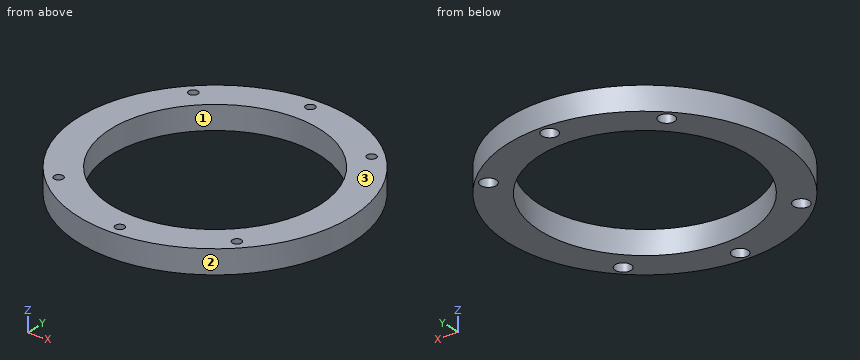
from build123d import *

# Parameters (mm, degrees)
CYLINDER057_R       = 87
CYLINDER057_DEPTH   = 15
CYLINDER058_R       = 66.5
CYLINDER058_DEPTH   = 15
HOLE019_D           = 5.8
HOLE019_DEPTH       = 25
HOLE019_CBORE_D     = 10
HOLE019_CBORE_DEPTH = 5.4


with BuildPart() as part:
    # Cylinder057 → Cylinder057 (join)
    with BuildSketch(Plane.XY):
        Circle(CYLINDER057_R)
    extrude(amount=CYLINDER057_DEPTH)

    # Cylinder058 → Cylinder058 (cut)
    with BuildSketch(Plane.XY):
        Circle(CYLINDER058_R)
    extrude(amount=CYLINDER058_DEPTH, mode=Mode.SUBTRACT)

    # Hole019
    with Locations(Plane(origin=(0, 0, 0), x_dir=(1, 0, 0), z_dir=(0, 0, -1))):
        with Locations((0, -79.861908), (56.470897, -56.470897), (56.470897, 56.470897), (0, 79.861908), (-56.470897, 56.470897), (-56.470897, -56.470897), (0, -79.861908)):
            CounterBoreHole(HOLE019_D / 2, HOLE019_CBORE_D / 2, HOLE019_CBORE_DEPTH, depth=HOLE019_DEPTH)


with BuildPart() as part_1:
    # Body055 placement: moved
    add(part.part.moved(Location((0, 0, -105))))


solid = part_1.part
CAD build for the part. Positions are in the model's coordinates, mm. Face numbers are marked on the shaded views. Round coordinates to 2 decimals unless told otherwise and drop trailing zeros. Order: outer loops, then holes, each group sorted by start corner. A loop starts at its lowest first (then second) coordinate and runs counter-clockwise, first axis right, second up. Notation, with made-up numbers: (55, 41) -> (85, 41) arc R19 ccw to (85, 76) -> close; hole circle Ø10 at (25.5, 0). An arc over 180 degrees is marked (long way). Write item = value, one per line. Start each with the question number.
(1) Pull direction X, two halves, no side cores. Call the marked faces 1, 2 and 3: released by +X, released by -X, zero draft, split by the parting line, or undercut.
(2) Probe line 1 (Y direction, x = 0, z = -101.55); line 2 (Y direction, x = 0, z = -94.25); line 3 (X direction, y = -0.5, z = -93.5). List the from-to ranges inside material, lowest first. Write a range as [from, to].
(3) Cut at A-A, the plane x = 0. List the corners of the cut face in (y, z).
(4) Cut at C-C, the plane x = 23.5. List the corners of the cut face in (y, z), then the cut area to 3 significant figures.
(5) Pin check, flat tips, straight feed: P1, Ø1.5, axis at y = 12, z = -99.5, coming from the -X side; P2, Ø3.5, axis at x = 0, y = -79.86, coming from the -Z side; P3, Ø5, axis at x = 54.5, y = 55.5, coming from the -Z side; P4, Ø8, axis at x = 49.5, z = -93, coming from the -Y side. Stop position of each tip, or through.
(6) Cut at B-B, the plane y = 0. List the corners of the cut face in (x, z).
(7) Cut at D-D, the plane z = -101.75. List the corners of the cut face in (x, y), then the cut area to 3 significant figures.
Model answer:
q1.face_1 = undercut
q1.face_2 = split by the parting line
q1.face_3 = zero draft
q2.line_1 = [-87, -84.86], [-74.86, -66.5], [66.5, 74.86], [84.86, 87]
q2.line_2 = [-87, -82.76], [-76.96, -66.5], [66.5, 76.96], [82.76, 87]
q2.line_3 = [-87, -66.5], [66.5, 87]
q3.outline = (-87, -105) -> (-84.86, -105) -> (-84.86, -99.6) -> (-82.76, -99.6) -> (-82.76, -90) -> (-87, -90) -> close; (-76.96, -99.6) -> (-74.86, -99.6) -> (-74.86, -105) -> (-66.5, -105) -> (-66.5, -90) -> (-76.96, -90) -> close; (66.5, -105) -> (74.86, -105) -> (74.86, -99.6) -> (76.96, -99.6) -> (76.96, -90) -> (66.5, -90) -> close; (82.76, -99.6) -> (84.86, -99.6) -> (84.86, -105) -> (87, -105) -> (87, -90) -> (82.76, -90) -> close
q4.outline = (-83.77, -105) -> (-62.21, -105) -> (-62.21, -90) -> (-83.77, -90) -> close; (62.21, -105) -> (83.77, -105) -> (83.77, -90) -> (62.21, -90) -> close
q4.area = 647 mm2
q5.P1 = -86.27
q5.P2 = through
q5.P3 = -99.6
q5.P4 = -74.15
q6.outline = (-87, -105) -> (-66.5, -105) -> (-66.5, -90) -> (-87, -90) -> close; (66.5, -105) -> (87, -105) -> (87, -90) -> (66.5, -90) -> close
q7.outline = circle Ø174 at (0, 0); hole circle Ø133 at (0, 0); hole circle Ø10 at (-56.47, -56.47); hole circle Ø10 at (-56.47, 56.47); hole circle Ø10 at (0, -79.86); hole circle Ø10 at (0, 79.86); hole circle Ø10 at (56.47, -56.47); hole circle Ø10 at (56.47, 56.47)
q7.area = 9,410 mm2
